```python
from build123d import *

# Parameters (mm, degrees)
F0_R     = 45
F0_R_2   = 3
F1_DEPTH = 6
F2_DEPTH = 6
F3_DEPTH = 6
F4_R     = 3.7046824746
F4_R_2   = 3.6592764752
F4_R_3   = 3.6139160681
F4_R_4   = 3.8159810343
F5_DEPTH = 2
F6_DEPTH = 2


with BuildPart() as f1:
    # F0 (on Top) → F1 (new body)
    with BuildSketch(Plane.XY):
        with Locations((0.0959349175, -0.0479674588)):
            Circle(F0_R)
        with Locations((0.0959349175, -39.9090653906)):
            Circle(F0_R_2, mode=Mode.SUBTRACT)
        with Locations((-40.0529677669, -0.0479674588)):
            Circle(F0_R_2, mode=Mode.SUBTRACT)
        with BuildLine():
            ThreePointArc((27.4207573821, 21.8233397102), (33.1214461646, 11.5414935671), (35.0959349175, -0.0479674588))
            ThreePointArc((35.0959349175, -0.0479674588), (33.1214461646, -11.6374284846), (27.4207573821, -21.9192746278))
            ThreePointArc((27.4207573821, -21.9192746278), (24.533111856, -25.104391451), (21.2767449211, -27.9114433294))
            ThreePointArc((21.2767449211, -27.9114433294), (21.9273327718, -29.335683713), (22.1502168829, -30.8855378658))
            ThreePointArc((22.1502168829, -30.8855378658), (17.7806491067, -36.268113735), (11.6148994329, -33.0981332147))
            ThreePointArc((11.6148994329, -33.0981332147), (-0.8185531736, -35.0360184409), (-13.1337970765, -32.4512727125))
            ThreePointArc((-13.1337970765, -32.4512727125), (-20.8976351843, -34.6820549215), (-22.5115050489, -26.7669430784))
            ThreePointArc((-22.5115050489, -26.7669430784), (-24.9875791947, -24.4573369668), (-27.228887547, -21.9192746278))
            ThreePointArc((-27.228887547, -21.9192746278), (-34.5685439732, -4.8826239339), (-32.1705090074, 13.512143029))
            ThreePointArc((-32.1705090074, 13.512143029), (-29.9880933208, 17.8392135644), (-27.228887547, 21.8233397102))
            ThreePointArc((-27.228887547, 21.8233397102), (-24.2059494655, 25.1396964948), (-20.7835404411, 28.042022017))
            ThreePointArc((-20.7835404411, 28.042022017), (-18.6742910421, 35.8397549184), (-11.0663916751, 33.1243472787))
            ThreePointArc((-11.0663916751, 33.1243472787), (1.0160924151, 34.9399348816), (12.9864428976, 32.4917744581))
            ThreePointArc((12.9864428976, 32.4917744581), (19.1675795097, 35.4283855992), (23.4248644926, 30.0706193309))
            ThreePointArc((23.4248644926, 30.0706193309), (23.1684252605, 28.4107788343), (22.4230206839, 26.9057195095))
            ThreePointArc((22.4230206839, 26.9057195095), (25.0516084979, 24.4920886975), (27.4207573821, 21.8233397102))
        make_face(mode=Mode.SUBTRACT)
        with Locations((39.6692280968, -0.0479674588)):
            Circle(F0_R_2, mode=Mode.SUBTRACT)
        with Locations((0.0959349175, 40.1009352257)):
            Circle(F0_R_2, mode=Mode.SUBTRACT)
        with BuildLine():
            ThreePointArc((21.2767449211, -27.9114433294), (24.533111856, -25.104391451), (27.4207573821, -21.9192746278))
            Line((27.4207573821, -21.9192746278), (6.5959349175, -21.9192746278))
            ThreePointArc((6.5959349175, -21.9192746278), (0.0959349175, -28.4192746278), (-6.4040650825, -21.9192746278))
            Line((-6.4040650825, -21.9192746278), (-27.228887547, -21.9192746278))
            ThreePointArc((-27.228887547, -21.9192746278), (-24.9875791947, -24.4573369668), (-22.5115050489, -26.7669430784))
            ThreePointArc((-22.5115050489, -26.7669430784), (-16.3594497928, -24.7438409966), (-12.5466565285, -29.9786603278))
            ThreePointArc((-12.5466565285, -29.9786603278), (-12.6954544679, -31.2493438081), (-13.1337970765, -32.4512727125))
            ThreePointArc((-13.1337970765, -32.4512727125), (-0.8185531736, -35.0360184409), (11.6148994329, -33.0981332147))
            ThreePointArc((11.6148994329, -33.0981332147), (14.0488297169, -26.0396339447), (21.2767449211, -27.9114433294))
        make_face()
        with BuildLine():
            Line((6.5959349175, 21.8233397102), (27.4207573821, 21.8233397102))
            ThreePointArc((27.4207573821, 21.8233397102), (25.0516084979, 24.4920886975), (22.4230206839, 26.9057195095))
            ThreePointArc((22.4230206839, 26.9057195095), (15.1231755594, 25.3376985497), (12.9864428976, 32.4917744581))
            ThreePointArc((12.9864428976, 32.4917744581), (1.0160924151, 34.9399348816), (-11.0663916751, 33.1243472787))
            ThreePointArc((-11.0663916751, 33.1243472787), (-10.7366623963, 32.0675422609), (-10.6252480106, 30.966113608))
            ThreePointArc((-10.6252480106, 30.966113608), (-14.6038355694, 25.6807277012), (-20.7835404411, 28.042022017))
            ThreePointArc((-20.7835404411, 28.042022017), (-24.2059494655, 25.1396964948), (-27.228887547, 21.8233397102))
            Line((-27.228887547, 21.8233397102), (-6.4040650825, 21.8233397102))
            ThreePointArc((-6.4040650825, 21.8233397102), (0.0959349175, 28.3233397102), (6.5959349175, 21.8233397102))
        make_face()
    extrude(amount=F1_DEPTH)

    # F0 (on Top) → F2 (join)
    with BuildSketch(Plane.XY):
        with BuildLine():
            Line((27.4207573821, 13.512143029), (27.4207573821, 21.8233397102))
            Line((27.4207573821, 21.8233397102), (6.5959349175, 21.8233397102))
            ThreePointArc((6.5959349175, 21.8233397102), (0.0959349175, 15.3233397102), (-6.4040650825, 21.8233397102))
            Line((-6.4040650825, 21.8233397102), (-27.228887547, 21.8233397102))
            Line((-27.228887547, 21.8233397102), (-27.228887547, 13.512143029))
            Line((-27.228887547, 13.512143029), (27.4207573821, 13.512143029))
        make_face()
    extrude(amount=F2_DEPTH)

    # F0 (on Top) → F3 (join)
    with BuildSketch(Plane.XY):
        with BuildLine():
            Line((6.5959349175, -21.9192746278), (27.4207573821, -21.9192746278))
            Line((27.4207573821, -21.9192746278), (27.4207573821, -13.512143029))
            Line((27.4207573821, -13.512143029), (-27.228887547, -13.512143029))
            Line((-27.228887547, -13.512143029), (-27.228887547, -21.9192746278))
            Line((-27.228887547, -21.9192746278), (-6.4040650825, -21.9192746278))
            ThreePointArc((-6.4040650825, -21.9192746278), (0.0959349175, -15.4192746278), (6.5959349175, -21.9192746278))
        make_face()
    extrude(amount=F3_DEPTH)

    # F4 (on face) → F5 (join)
    with BuildSketch(Plane.XY.offset(6)):
        with Locations((-40.0529677669, -0.0479674588)):
            Circle(F4_R)
        with Locations((0.0959349175, 40.1009352257)):
            Circle(F4_R_2)
        with Locations((39.6692280968, -0.0479674588)):
            Circle(F4_R_3)
        with Locations((0.0959349175, -39.9090653906)):
            Circle(F4_R_4)
    extrude(amount=-F5_DEPTH)

    # F4 (on face) → F6 (join)
    with BuildSketch(Plane.XY.offset(6)):
        with Locations((-40.0529677669, -0.0479674588)):
            Circle(F4_R)
        with Locations((0.0959349175, 40.1009352257)):
            Circle(F4_R_2)
        with Locations((39.6692280968, -0.0479674588)):
            Circle(F4_R_3)
        with Locations((0.0959349175, -39.9090653906)):
            Circle(F4_R_4)
    extrude(amount=-F6_DEPTH)


solid = f1.part
```
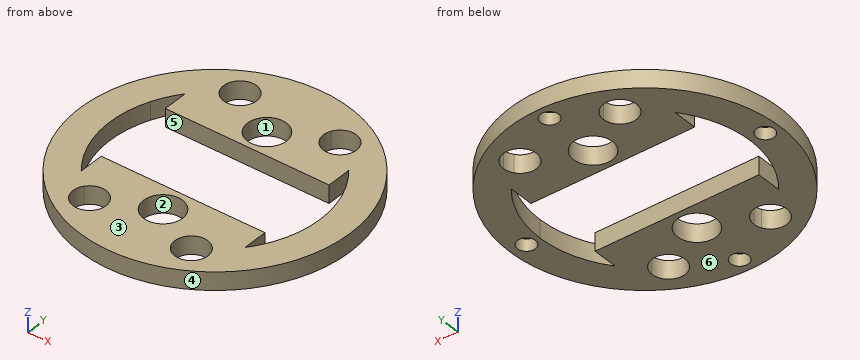
CAD build for the part. Positions are in the model's coordinates, mm. Face numbers are marked on the shaded views. A direction names the side the tool comes from. Coordinates: 2 decimals unless noted, no trailing zeros. Write each loop counter-clockwise with the first axis right and the second up, starting at its lowest first coordinate (ties: lowest second). Pieces come first, ordered by that corner, then holes.
(1) Cut at B-B, the plane y = 18.5. List the corners of the cut face in (x, z), and give its area (3 significant figures).
(2) Cut at C-C, the plane z = 1.6. Count the separate pieces of the cut face and the enclosed holes in it, and give its area (3 significant figures).
(3) 3-axis set-ups, long thin cutter, end or side, ignore diameter. For the marked faces 5 and 6: which of +Z, -Z, +X, -X, +Y, -Y reach the whole face in a straight line?
(4) Cut at A-A, the plane x = -15. List the corners of the cut face in (y, z), and give its area (3 significant figures).
(5) Two-plate mould, pull along X, no slides. Class the marked faces 1, 2, 3 and 4: +X half, -X half, draft (parallel to the pull), parting line (faces both ways), or undercut.
(6) Cut at D-D, the plane y = -8.5. List the corners of the cut face in (x, z), and give its area (3 significant figures).
(7) Drill centre lines: probe 1 along Y at (x, z) = (0.5, 5.1); probe 2 along X at (y, z) = (-16.5, 5.35); probe 3 along X at (y, z) = (31.5, 4.5). Where is each one in solid material? Low to high.
(8) Flat gauge pins, fed straight in: pin 1 (1.5 mm diameter, centred on x = -33, y = -3, fed in from +Z); pin 2 (1.8 mm diameter, centred on y = 16.5, z = 3, fed in from +X); pin 3 (2 mm diameter, centred on y = -3, z = 2, fed in from +X); pin 4 (1 mm diameter, centred on y = -16.5, z = 4, fed in from -X). Where does each tip first touch, or does it go through?
Geometry says:
1. outline: (-40.9, 0) - (-29.59, 0) - (-29.59, 6) - (-40.9, 6) - close; (-27.23, 0) - (-5.49, 0) - (-5.49, 6) - (-27.23, 6) - close; (5.68, 0) - (27.42, 0) - (27.42, 6) - (5.68, 6) - close; (29.78, 0) - (41.1, 0) - (41.1, 6) - (29.78, 6) - close
1. area: 397 mm2
2. separate pieces: 1
2. enclosed holes: 11
2. area: 3,670 mm2
3. face 5: +Z, -Z
3. face 6: -Z, +X, -X, +Y, -Y
4. outline: (-42.44, 0) - (-34.56, 0) - (-34.56, 6) - (-42.44, 6) - close; (-25.4, 0) - (-13.51, 0) - (-13.51, 6) - (-25.4, 6) - close; (13.51, 0) - (25.58, 0) - (25.58, 6) - (13.51, 6) - close; (36.35, 0) - (42.34, 0) - (42.34, 6) - (36.35, 6) - close
4. area: 227 mm2
5. face 1: undercut
5. face 2: undercut
5. face 3: draft
5. face 4: parting line
6. outline: (-44.1, 0) - (-33.87, 0) - (-33.87, 6) - (-44.1, 6) - close; (34.06, 0) - (44.3, 0) - (44.3, 6) - (34.06, 6) - close
6. area: 123 mm2
7. probe 1: y = -45.05 to -28.41, -15.43 to -13.51, 13.51 to 15.34, 28.31 to 44.95
7. probe 2: x = -41.79 to -30.8, -27.23 to -3.49, 3.69 to 27.42, 30.99 to 41.98
7. probe 3: x = -31.99 to -21.6, -10.65 to 12.61, 23.24 to 32.19
8. pin 1: passes through
8. pin 2: stops at x = 42.29
8. pin 3: stops at x = 45.05
8. pin 4: stops at x = -41.98
